```python
from build123d import *

# Parameters (mm, degrees)
SKETCH004_R  = 1.75
PAD005_DEPTH = 2
SKETCH002_W  = 6
SKETCH002_H  = 6
PAD003_DEPTH = 0.2


with BuildPart() as body004:
    # Sketch004 → Pad005 (new body)
    with BuildSketch(Plane.XY):
        Circle(SKETCH004_R)
    extrude(amount=PAD005_DEPTH)


with BuildPart() as body004_1:
    # Body004 placement: moved
    add(body004.part.moved(Location((0, 0, 7))))


with BuildPart() as cut:
    # Sketch002 → Pad003 (new body)
    with BuildSketch(Plane.XY):
        Rectangle(SKETCH002_W, SKETCH002_H)
    extrude(amount=PAD003_DEPTH)


with BuildPart() as cut_1:
    # Body002 placement: moved
    add(cut.part.moved(Location((0, 0, 7))))

    # Cut: cut Body004
    add(body004_1.part, mode=Mode.SUBTRACT)


solid = cut_1.part
```
For this review, take the finished solid that the model builds, in its own axes (mm). Coordinates: 2 decimals unless noted, no trailing zeros. Order: outer loops, then holes, each group sorted by start corner. A loop starts at its lowest first (then second) coordinate and runs counter-clockwise, first axis right, second up. Notation, with made-up numbers: (73, 35.25) -> (129, 35.25) arc R30 cw to (129, 67.25) -> close; hole circle Ø10 at (35, 36.5). An arc over 180 degrees is marked (long way). Answer as CSV lines item,"result".
Q1. We need section A-A (y = 0). State the section outline as (x, z) points.
Model answer:
outline,"(-3, 7) -> (-1.75, 7) -> (-1.75, 7.2) -> (-3, 7.2) -> close; (1.75, 7) -> (3, 7) -> (3, 7.2) -> (1.75, 7.2) -> close"
Q2. Clearance check with a flat-ended pin moving along its axis: pin 1 Ø3 at (x, y) = (0, 0) entering from -Z. State where the tip first meets the part, or that it passes through.
Model answer:
pin 1,"passes through"
Q3. Wall thickness on line 1 along Y through (x, z) = (0, 7.15); line 2 along Y through (x, z) = (-1.1, 7.1): over which ranges is each line inside the solid? List them lowest first. Write a range as [from, to].
Model answer:
line 1,"y = [-3, -1.75], [1.75, 3]"
line 2,"y = [-3, -1.36], [1.36, 3]"
Q4. We need section C-C (z = 7.15). State the section outline as (x, y) points.
Model answer:
outline,"(-3, -3) -> (3, -3) -> (3, 3) -> (-3, 3) -> close; hole circle Ø3.5 at (0, 0)"
